```python
from build123d import *

# Parameters (mm, degrees)
SKETCH1_R           = 2.5
BOSS_EXTRUDE1_DEPTH = 3.5
FILLET1_R           = 3
SKETCH2_W           = 75.5
SKETCH2_H           = 30.382012963
SKETCH2_R           = 4.125
SKETCH2_R_2         = 2.5
BOSS_EXTRUDE2_DEPTH = 3.5
SKETCH2_4_W         = 8.340351234
SKETCH2_4_H         = 13.691006481
SKETCH2_4_R         = 2.5
SKETCH2_4_H_2       = 13.691006482
BOSS_EXTRUDE3_DEPTH = 16
FILLET2_R           = 3
FILLET3_R           = 3
SKETCH2_7_W         = 8.340351234
SKETCH2_7_H         = 3
BOSS_EXTRUDE5_DEPTH = 12


with BuildPart() as part:
    # Sketch1 → Boss-Extrude1 (new body)
    with BuildSketch(Plane.XY):
        Polygon((-32.756938656, -9), (36.41997588, -9), (56.136580269, 17.570938838), (56.136580269, 50.908965344), (1.831518612, 50.908965344), align=None)
        with Locations((-17.168481388, 0)):
            Circle(SKETCH1_R, mode=Mode.SUBTRACT)
        with Locations((20.831518612, 0)):
            Circle(SKETCH1_R, mode=Mode.SUBTRACT)
        with Locations((1.831518612, 32.908965344)):
            Circle(SKETCH1_R, mode=Mode.SUBTRACT)
    extrude(amount=BOSS_EXTRUDE1_DEPTH)

    # Fillet1
    fillet1_edges = [part.edges().sort_by_distance(p)[0] for p in [
        (36.41997588, -9, 1.75),
        (-32.756938656, -9, 1.75),
        (1.831518612, 50.908965344, 1.75),
    ]]
    fillet(fillet1_edges, radius=FILLET1_R)

    # Sketch2 → Boss-Extrude2 (add)
    with BuildSketch(Plane(origin=(0, 0, 0), x_dir=(-1, 0, 0), z_dir=(0, 0, -1))):
        with Locations((-17.421869846, 32.908965344)):
            Rectangle(SKETCH2_W, SKETCH2_H)
        with Locations((-1.831518612, 32.908965344)):
            Circle(SKETCH2_R, mode=Mode.SUBTRACT)
        with Locations((16.168481388, 40.908965344)):
            Circle(SKETCH2_R_2, mode=Mode.SUBTRACT)
        with Locations((16.168481388, 24.908965344)):
            Circle(SKETCH2_R_2, mode=Mode.SUBTRACT)
        with Locations((-50.831518612, 24.908965344)):
            Circle(SKETCH2_R_2, mode=Mode.SUBTRACT)
        with Locations((-50.831518612, 40.908965344)):
            Circle(SKETCH2_R_2, mode=Mode.SUBTRACT)
    extrude(amount=-BOSS_EXTRUDE2_DEPTH)

    # Sketch2<4> → Boss-Extrude3 (add)
    # profile 1 of 2: a face of its own
    with BuildSketch(Plane(origin=(0, 0, 0), x_dir=(-1, 0, 0), z_dir=(0, 0, -1))):
        with Locations((-51.001694229, 41.254468585)):
            Rectangle(SKETCH2_4_W, SKETCH2_4_H)
        with Locations((-50.831518612, 40.908965344)):
            Circle(SKETCH2_4_R, mode=Mode.SUBTRACT)
    # profile 2 of 2: a face of its own
    with BuildSketch(Plane(origin=(0, 0, 0), x_dir=(-1, 0, 0), z_dir=(0, 0, -1))):
        with Locations((-51.001694229, 24.563462103)):
            Rectangle(SKETCH2_4_W, SKETCH2_4_H_2)
        with Locations((-50.831518612, 24.908965344)):
            Circle(SKETCH2_4_R, mode=Mode.SUBTRACT)
    extrude(amount=BOSS_EXTRUDE3_DEPTH)

    # Fillet2
    # the kernel refuses this fillet: 3 mm, written as the material it adds along each edge
    with BuildSketch(Plane(origin=(-17.331317914, 17.717958862, 0), x_dir=(-0.4999999999999997, -0.8660254037844388, 0), z_dir=(0, 0, 1))) as fillet2_piece_1:
        with BuildLine():
            CenterArc((4.470985889, -3), FILLET2_R, 90, 82.247461928)
            Line((1.49840612, -2.59531553), (1.438954525, -2.587221841))
            ThreePointArc((1.438954525, -2.587221841), (0.697241536, -1.327657765), (-0.051961524, -0.03))
            Line((-0.051961524, -0.03), (0, 0.06))
            Line((0, 0.06), (4.470985889, 0.06))
            Line((4.470985889, 0.06), (4.470985889, 0))
        make_face()
    extrude(amount=3.5)

    # Fillet3
    fillet3_edges = [part.edges().sort_by_distance(p)[0] for p in [
        (-20.328130154, 48.099971825, 1.75),
        (56.136580269, 50.908965344, 1.75),
        (56.136580269, 17.570938838, 1.75),
    ]]
    fillet(fillet3_edges, radius=FILLET3_R)

    # Sketch2<7> → Boss-Extrude5 (add)
    with BuildSketch(Plane(origin=(0, 0, 0), x_dir=(-1, 0, 0), z_dir=(0, 0, -1))):
        with Locations((-51.001694229, 32.908965344)):
            Rectangle(SKETCH2_7_W, SKETCH2_7_H)
    extrude(amount=BOSS_EXTRUDE5_DEPTH)


solid = part.part
```
Read the model definition and answer for the solid it produces. Units are mm, in the model's axes. A direction names the side the tool comes from. Give positions to 0.01 mm unless a question says otherwise; leave off trailing zeros. Order: outer loops, then holes, each group sorted by start corner. A loop starts at its lowest first (then second) coordinate and runs counter-clockwise, first axis right, second up. Notation, with made-up numbers: (74, 9) -> (80, 9) arc R16 cw to (80, 32) -> close; hole circle Ø1 at (13.25, 42.25). An arc over 180 degrees is marked (long way). Write item = value, one per line.
1. A cutting plane is placed at B-B, the plane y = 0. Write down the section's boundary in (x, z), and give its area (3 significant figures).
Numbers:
outline = (-27.56, 0) -> (-19.67, 0) -> (-19.67, 3.5) -> (-27.56, 3.5) -> close; (-14.67, 0) -> (18.33, 0) -> (18.33, 3.5) -> (-14.67, 3.5) -> close; (23.33, 0) -> (43.1, 0) -> (43.1, 3.5) -> (23.33, 3.5) -> close
area = 212 mm²
2. For faces 4 (the face through (12, 21, 3.5)), 5 (the face through (55.172, 33, -8)), 6 (the face through (48.447, 41.66, -7.888)), 7 (the face through (46.832, 33, -8)), 8 (the face through (51, 33, -12)), determine the directions among +Z, -Z, +X, -X, +Y, -Y from which every point of the face is accessible in a straight line to the end or side of a thin tool.
Numbers:
face_4 = +Z, +X, -X, +Y, -Y
face_5 = -Z, +X, +Y, -Y
face_6 = -Z
face_7 = -Z, -X, +Y, -Y
face_8 = -Z, +X, -X
3. Given pin 1 (2.5 mm diameter, centred on x = 52, z = -4, fed in from -Y); pin 2 (1.5 mm diameter, centred on x = 51, y = 26, fed in from -Z); pin 3 (4.5 mm diameter, centred on x = 20.83, y = 0, fed in from -Z); pin 4 (1.2 mm diameter, centred on x = 49.5, z = -14, fed in from +Y), each flat-ended and moving along its own axis, determine where each tip first touches the part or whether it passes through.
Numbers:
pin_1 = 17.72
pin_2 = 0
pin_3 = through
pin_4 = 48.1
4. A cutting plane is placed at A-A, the plane z = -13.25. Write down the section's boundary in (x, y).
Numbers:
outline = (46.83, 17.72) -> (55.17, 17.72) -> (55.17, 31.41) -> (46.83, 31.41) -> close; (46.83, 34.41) -> (55.17, 34.41) -> (55.17, 48.1) -> (46.83, 48.1) -> close; hole circle Ø5 at (50.83, 24.91); hole circle Ø5 at (50.83, 40.91)
5. A cutting plane is placed at D-D, the plane z = -6. Write down the section's boundary in (x, y), and give its area (3 significant figures).
Numbers:
outline = (46.83, 17.72) -> (55.17, 17.72) -> (55.17, 48.1) -> (46.83, 48.1) -> close; hole circle Ø5 at (50.83, 24.91); hole circle Ø5 at (50.83, 40.91)
area = 214 mm²
6. The mould has two halves that part along Y. Classify faces 1 (the face through (3, -9, 2)), 2 (the face through (-8, 48.1, 2)), 3 (the face through (51, 41, 0)): +Y half, -Y half, draft (parallel to the pull), parting line (faces both ways), or undercut.
Numbers:
face_1 = -Y half
face_2 = +Y half
face_3 = undercut
7. A cutting plane is placed at C-C, the plane x = 17. Write down the section's boundary in (y, z), and give its area (3 significant figures).
Numbers:
outline = (-9, 0) -> (50.91, 0) -> (50.91, 3.5) -> (-9, 3.5) -> close
area = 210 mm²
8. Straight lines are drawn through the part: line 1 along X through (y, z) = (41, -14.75); line 2 along Y through (x, z) = (52.5, -13.75); line 3 along Z through (x, y) = (-4, 37). For each, find the intervals that lie inside material, in ascending order.
Numbers:
line_1 = 46.83 to 48.33, 53.33 to 55.17
line_2 = 17.72 to 23.05, 26.77 to 31.41, 34.41 to 39.05, 42.77 to 48.1
line_3 = 0 to 3.5
